Work out the finished part from the listing and answer in its coordinate system (mm). Round coordinates to 2 decimals unless told otherwise and drop trailing zeros. Write each loop counter-clockwise with the first axis right and the second up, starting at its lowest first coordinate (ties: lowest second). Pieces come first, ordered by that corner, then holes.
1. Determine the mould class of faces 1 (the face through (-4.26, -45.185, 2.465)), 2 (the face through (-3, 3, 5)), 3 (the face through (-41.19, -185.48, 2.46)) for opening direction X: pulls with the +X half, pulls with the -X half, needs draft (parallel to the pull), parting line crosses it, or undercut.
2. Straight lines are drawn through the part: probe 1 along Y at (x, z) = (0, 2.4); probe 2 along Y at (x, z) = (45.5, 3.5); probe 3 along Y at (x, z) = (-50.5, 1.3). For each, find the intervals that lie inside material, in ascending order.
3. Flat-ended cylindrical pins translate along their axes: pin 1 Ø7 at (x, y) = (30.78, 39.4) entering from +Z; pin 2 Ø2 at (y, z) = (148.5, 2.5) entering from +X; pin 3 Ø3 at (y, z) = (-117.5, 2.5) entering from -X; pin 4 Ø1.5 at (y, z) = (44, 2) entering from -X. Find the tip coordinate at first contact, or state that the pin passes through.
4. Find section C-C (z = 2.1). Count the separate pieces of the cut face and the enclosed holes in it, and give its area (3 significant figures).
5. Find section D-D (x = -119). Write down the section's boundary in (y, z), and give its area (3 significant figures).
6. Find section B-B (y = 25). Write down the section's boundary in (x, z), and give its area (3 significant figures).
7. Find section A-A (x = -39). Write down the section's boundary in (y, z), and give its area (3 significant figures).
```python
from build123d import *

# Parameters (mm, degrees)
SKETCH1_R           = 190
BOSS_EXTRUDE1_DEPTH = 5
SKETCH2_R           = 9
SKETCH2_R_2         = 6
CUT_EXTRUDE1_DEPTH  = 10


with BuildPart() as part:
    # Sketch1 → Boss-Extrude1 (new body)
    with BuildSketch(Plane.XY):
        Circle(SKETCH1_R)
    extrude(amount=BOSS_EXTRUDE1_DEPTH)

    # Sketch2 → Cut-Extrude1 (cut)
    with BuildSketch(Plane(origin=(0, 0, 0), x_dir=(-1, 0, 0), z_dir=(0, 0, -1))):
        with Locations((0, 50)):
            Circle(SKETCH2_R)
        with Locations((43.301270189, 25)):
            Circle(SKETCH2_R)
        with Locations((43.301270189, -25)):
            Circle(SKETCH2_R)
        with Locations((-30.783073766, 39.40053768)):
            Circle(SKETCH2_R_2)
        with Locations((-48.514786314, 12.09609478)):
            Circle(SKETCH2_R_2)
        with Locations((-45.677272882, -20.336832154)):
            Circle(SKETCH2_R_2)
        with Locations((-23.473578139, -44.147379643)):
            Circle(SKETCH2_R_2)
        with Locations((8.682408883, -49.240387651)):
            Circle(SKETCH2_R_2)
    extrude(amount=-CUT_EXTRUDE1_DEPTH, mode=Mode.SUBTRACT)


solid = part.part
```
Worked answers:
1. face 1: undercut
1. face 2: needs draft
1. face 3: parting line crosses it
2. probe 1: y = -190 to 41, 59 to 190
2. probe 2: y = -184.47 to -26.33, -14.34 to 6.91, 17.28 to 184.47
2. probe 3: y = -183.17 to -30.4, -19.6 to 19.6, 30.4 to 183.17
3. pin 1: passes through
3. pin 2: stops at x = 119.77
3. pin 3: stops at x = -150.48
3. pin 4: stops at x = -185.01
4. separate pieces: 1
4. enclosed holes: 8
4. area: 112,000 mm2
5. outline: (-148.12, 0) - (148.12, 0) - (148.12, 5) - (-148.12, 5) - close
5. area: 1,480 mm2
6. outline: (-188.35, 0) - (-52.3, 0) - (-52.3, 5) - (-188.35, 5) - close; (-34.3, 0) - (188.35, 0) - (188.35, 5) - (-34.3, 5) - close
6. area: 1,790 mm2
7. outline: (-185.95, 0) - (-32.91, 0) - (-32.91, 5) - (-185.95, 5) - close; (-17.09, 0) - (17.09, 0) - (17.09, 5) - (-17.09, 5) - close; (32.91, 0) - (185.95, 0) - (185.95, 5) - (32.91, 5) - close
7. area: 1,700 mm2
